Part print with two shaded views. Sizes in mm from the minimum x, y, z corner. A direction names the side the tool comes from. Round coordinates to 2 decimals unless told otherwise and drop trailing zeros. Order: outer loops, then holes, each group sorted by start corner. A loop starts at its lowest first (then second) coordinate and runs counter-clockwise, first axis right, second up. Notation, with made-up numbers: M 57,64 L 113,64 A22 cw 113,94 Z; hole C 0,-16.5 d5. An arc over 180 degrees is marked long. Put each result on its own line as item: value.
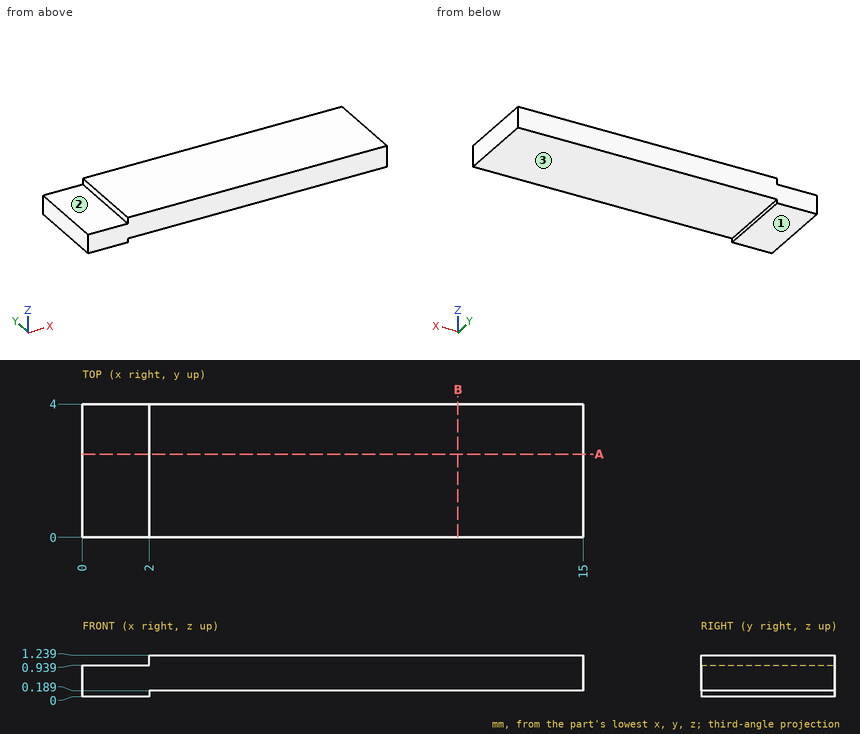
Item 1: Tool access for the marked faces 1, 2 and 3: list every direction of +Z, -Z, +X, -X, +Y, -Y with a clear straight run to the whole face (end or side of a thin tool).
Answers below:
face 1: -Z, +X, -X, +Y, -Y
face 2: +Z, -X, +Y, -Y
face 3: -Z, +X, +Y, -Y
Item 2: Band-saw the part on B-B on x = 11.25. Give the cut face in (y, z).
Answers below:
outline: M 0,0.19 L 4,0.19 L 4,1.24 L 0,1.24 Z
Item 3: Probe line 1 along X through (y, z) = (0.4, 1.15); line 2 along X through (y, z) = (0.2, 0.1); line 3 along Z through (x, y) = (13.5, 0.75). List the from-to ranges inside material, lowest first. Write a range as [from, to].
Answers below:
line 1: [2, 15]
line 2: [0, 2]
line 3: [0.19, 1.24]
Item 4: Pin check, flat tip, straight feed: P1, Ø2, axis at x = 1.5, y = 1.5, coming from the +Z side. Stop position of the tip, or through.
Answers below:
P1: z = 1.24
Item 5: Band-saw the part on A-A on y = 2.5. Give the cut face in (x, z).
Answers below:
outline: M 0,0 L 2,0 L 2,0.19 L 15,0.19 L 15,1.24 L 2,1.24 L 2,0.94 L 0,0.94 Z
